Geometry check sheet. Reference: the model listing, model coordinates, mm. Face numbers are marked on the shaded views. A direction names the side the tool comes from. Round coordinates to 2 decimals unless told otherwise and drop trailing zeros. Write each loop counter-clockwise with the first axis right and the second up, starting at its lowest first coordinate (ties: lowest second). Pieces come first, ordered by that corner, then holes. Notation, with made-up numbers: (6, 62.5) - (24, 62.5) arc R24 cw to (24, 95.5) - close; hole circle Ø6 at (12.25, -13.5). An arc over 180 degrees is marked (long way). Return JSON: item names as keys, results as strings. Group by question number.
from build123d import *

# Parameters (mm, degrees)
SKETCH1_R           = 5
BOSS_EXTRUDE1_DEPTH = 19
SKETCH2_R           = 4
BOSS_EXTRUDE2_DEPTH = 15
BOSS_EXTRUDE3_START = -53
SKETCH2_2_R         = 4
BOSS_EXTRUDE3_DEPTH = 15
CHAMFER2_SIZE       = 0.5
SKETCH5_R           = 2.6
BOSS_EXTRUDE4_DEPTH = 10
SKETCH7_R           = 2.6
BOSS_EXTRUDE5_DEPTH = 10


# Read off the part's stored shape, not the designer's step: M5 Machine Threads Stud3, M5 Machine Threads Stud4
with BuildPart() as part:
    # Sketch1 → Boss-Extrude1 (new, symmetric)
    with BuildSketch(Plane(origin=(0, 0, 0), x_dir=(1, 0, 0), z_dir=(0, 1, 0))):
        with Locations(Location((0, 0, 0), (0, 0, 270))):
            Circle(SKETCH1_R)
    extrude(amount=BOSS_EXTRUDE1_DEPTH, both=True)

    # Sketch2 → Boss-Extrude2 (add)
    with BuildSketch(Plane(origin=(0, 19, 0), x_dir=(1, 0, 0), z_dir=(0, 1, 0))):
        with Locations(Location((0, 0, 0), (0, 0, 270))):
            Circle(SKETCH2_R)
    extrude(amount=BOSS_EXTRUDE2_DEPTH)

    # Sketch2<2> → Boss-Extrude3 (add)
    with BuildSketch(Plane(origin=(0, 19, 0), x_dir=(1, 0, 0), z_dir=(0, 1, 0)).offset(BOSS_EXTRUDE3_START)):
        with Locations(Location((0, 0, 0), (0, 0, 270))):
            Circle(SKETCH2_2_R)
    extrude(amount=BOSS_EXTRUDE3_DEPTH)

    # Chamfer2
    chamfer2_edges = [part.edges().sort_by_distance(p)[0] for p in [
        (0, -34, -4),
        (0, -19, -4),
        (0, -19, -5),
        (0, 19, -5),
        (0, 34, -4),
    ]]
    chamfer(chamfer2_edges, length=CHAMFER2_SIZE - 0.0001)  # a hair under: the kernel refuses the full size

    # Sketch5 → Boss-Extrude4 (add)
    with BuildSketch(Plane.XZ.offset(34)):
        with Locations(Location((0, 0, 0), (0, 0, 270))):
            Circle(SKETCH5_R)
    extrude(amount=BOSS_EXTRUDE4_DEPTH)

    # M5 Machine Threads Stud3 outline → M5 Machine Threads Stud3 (revolve, cut)
    with BuildSketch(Plane.XY):
        with BuildLine():
            Line((2.6, -44), (2.6, -34))
            Line((2.6, -34), (2.4, -34))
            ThreePointArc((2.4, -34), (2.117157288, -34.117157288), (2, -34.4))
            Line((2, -34.4), (2, -35.1))
            ThreePointArc((2, -35.1), (2.013629669, -35.203527618), (2.053589838, -35.3))
            Line((2.053589838, -35.3), (2.5, -36.073205081))
            Line((2.5, -36.073205081), (2.5, -43.555))
            Line((2.5, -43.555), (2.055, -44))
            Line((2.055, -44), (2.6, -44))
        make_face()
    revolve(axis=Axis((0, 0, 0), (0, 1, 0)), mode=Mode.SUBTRACT)

    # Sketch7 → Boss-Extrude5 (add)
    with BuildSketch(Plane(origin=(0, 34, 0), x_dir=(1, 0, 0), z_dir=(0, 1, 0))):
        with Locations(Location((0, 0, 0), (0, 0, 270))):
            Circle(SKETCH7_R)
    extrude(amount=BOSS_EXTRUDE5_DEPTH)

    # M5 Machine Threads Stud4 outline → M5 Machine Threads Stud4 (revolve, cut)
    with BuildSketch(Plane.XY):
        with BuildLine():
            Line((2.6, 44), (2.055, 44))
            Line((2.055, 44), (2.5, 43.555))
            Line((2.5, 43.555), (2.5, 36.073205081))
            Line((2.5, 36.073205081), (2.053589838, 35.3))
            ThreePointArc((2.053589838, 35.3), (2.013629669, 35.203527618), (2, 35.1))
            Line((2, 35.1), (2, 34.4))
            ThreePointArc((2, 34.4), (2.117157288, 34.117157288), (2.4, 34))
            Line((2.4, 34), (2.6, 34))
            Line((2.6, 34), (2.6, 44))
        make_face()
    revolve(axis=Axis((0, 0, 0), (0, 1, 0)), mode=Mode.SUBTRACT)


solid = part.part
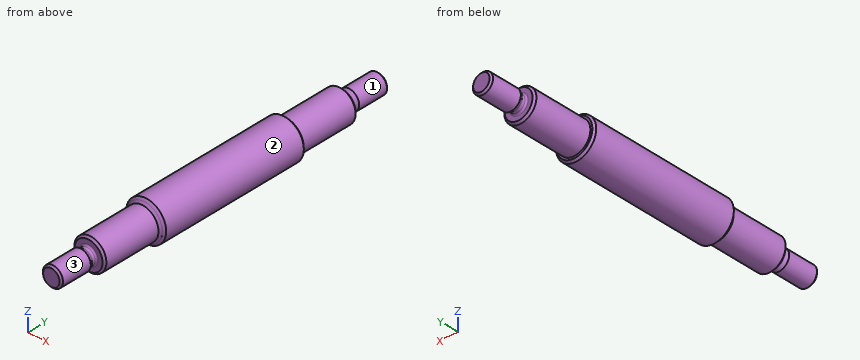
1. Tool access check on the marked faces 1, 2 and 3. Record the directions out of +Z, -Z, +X, -X, +Y, -Y that give a thin tool (end or side, any length) a straight path to the whole face; none if there is none.
2. Material ranges on line 1 along Y through (x, z) = (2.25, 1.5); line 2 along X through (y, z) = (28.5, 0); line 3 along Y through (x, z) = (-4, 2.25), recorded low to high.
3. Depth check by flat-ended pin: pin 1 Ø3 at (x, y) = (0, 34.5) entering from +Z; pin 2 Ø2 at (x, y) = (2.5, 12) entering from +Z; pin 3 Ø1 at (x, y) = (2.5, 14) entering from -Z. Enter the tip coordinate at first touch or a pass-through.
4. Section check A-A (y = 9.5). Enter the section's corners in (x, z), and give its area (3 significant figures).
Result sheet:
{
 "1": {"face 1": "+Y", "face 2": "+Y, -Y", "face 3": "-Y"},
 "2": {"line 1": "y = -34 to 34", "line 2": "x = -4 to 4", "line 3": "y = -18.91 to 18.91"},
 "3": {"pin 1": "stops at z = 4", "pin 2": "stops at z = 4.77", "pin 3": "stops at z = -4.58"},
 "4": {"outline": "circle Ø10 at (0, 0)", "area": "78.5 mm²"}
}
